The model under review builds one solid part; all positions refer to its coordinate system, in mm. Coordinates: 2 decimals unless noted, no trailing zeros. Use CSV: the item, a comma, the result in double quotes. Start each with the question number.
1. For L1, parallel to Y at x = 67, z = -9.5; L2, parallel to Z at x = 52.5, y = 10.5; L3, parallel to Z at x = 9, y = 17, list the stretches that pass through material, from the lowest coordinate up.
2. Draft analysis for pull direction X (two halves, no side actions). For faces 1 (the cylindrical face through (45.56, 3.01, -32.15)), 2 (the flat face through (0, 10, -17)), 3 (the cylindrical face through (88, 19, -18)), state which applies: +X half, -X half, draft (parallel to the pull), parting line (faces both ways), or undercut.
3. Clearance check with flat-ended pins moving along their axes: P1, Ø8, axis at x = 46, y = 16.5, coming from the +Z side; P2, Ø1, axis at x = 25, y = 11, coming from the -Z side. State where each tip first meets the part, or that it passes through.
from build123d import *

# Parameters (mm, degrees)
SKETCH1_W           = 90
SKETCH1_H           = 35
BOSS_EXTRUDE1_DEPTH = 20
FILLET1_R           = 10
FILLET2_R           = 5


with BuildPart() as part:
    # Sketch1 → Boss-Extrude1 (new body)
    with BuildSketch(Plane(origin=(0, 0, 0), x_dir=(1, 0, 0), z_dir=(0, 1, 0))):
        with Locations((45, 17.5)):
            Rectangle(SKETCH1_W, SKETCH1_H)
    extrude(amount=BOSS_EXTRUDE1_DEPTH)

    # Fillet1
    fillet1_edges = [part.edges().sort_by_distance(p)[0] for p in [
        (45, 20, -35),
        (45, 0, -35),
        (45, 0, 0),
        (45, 20, 0),
    ]]
    fillet(fillet1_edges, radius=FILLET1_R - 0.0001)  # a hair under: the kernel refuses the full size

    # Fillet2
    fillet2_edges = [part.edges().sort_by_distance(p)[0] for p in [
        (0, 20, -17.5),
        (90, 20, -17.5),
        (0, 0, -17.5),
        (0, 17.071097101, -2.928902899),
        (0, 2.928902899, -2.928902899),
        (0, 2.928902899, -32.071097101),
        (0, 17.071097101, -32.071097101),
        (90, 0, -17.5),
        (90, 17.071097101, -2.928902899),
        (90, 2.928902899, -2.928902899),
        (90, 2.928902899, -32.071097101),
        (90, 17.071097101, -32.071097101),
    ]]
    fillet(fillet2_edges, radius=FILLET2_R)


solid = part.part
Computed:
1,L1,"y = 0.01 to 19.99"
1,L2,"z = -34.99 to -0.01"
1,L3,"z = -32.14 to -2.86"
2,face 1,"draft"
2,face 2,"-X half"
2,face 3,"+X half"
3,P1,"stops at z = -0.32"
3,P2,"stops at z = -34.99"
